Geometry: see drawing. Coordinates: mm, zero at the bounding-box minimum. Give positions to 0.01 mm unless a question says otherwise; leave off trailing zeros. Write each loop counter-clockwise with the first axis right and the second up, starting at its lowest first coordinate (ties: lowest second). Pieces come first, ordered by that corner, then holes. Notation, with made-up numbers: (-4, 59.25) - (0, 59.25) arc R20 cw to (0, 73.25) - close; hole circle Ø3 at (46.5, -17). An arc over 180 degrees is marked (long way). Use a Markdown table: item, result. Add a question column.
1. Section query C-C, the plane x = 68. Return loops of the section in (y, z) (1 decimal).
2. Section query A-A, the plane x = 6.35. Return loops of the section in (y, z) (1 decimal).
3. Pin query (flat end, axial travel): pin 1 (0.5 mm diameter, centred on y = 3, z = 1, fed in from -X); pin 2 (1 mm diameter, centred on x = 30.5, y = 2.5, fed in from +Z); pin 3 (5 mm diameter, centred on x = 43, y = 1.5, fed in from -Z). Return the tip coordinate at first contact, or that it passes through.
4. Material intervals for probe 1 along Y at (x, z) = (6.35, 5) (1 decimal); probe 2 along X at (y, z) = (5, 3.75); probe 3 along Y at (x, z) = (77, 5) (1 decimal), sorted ascending.
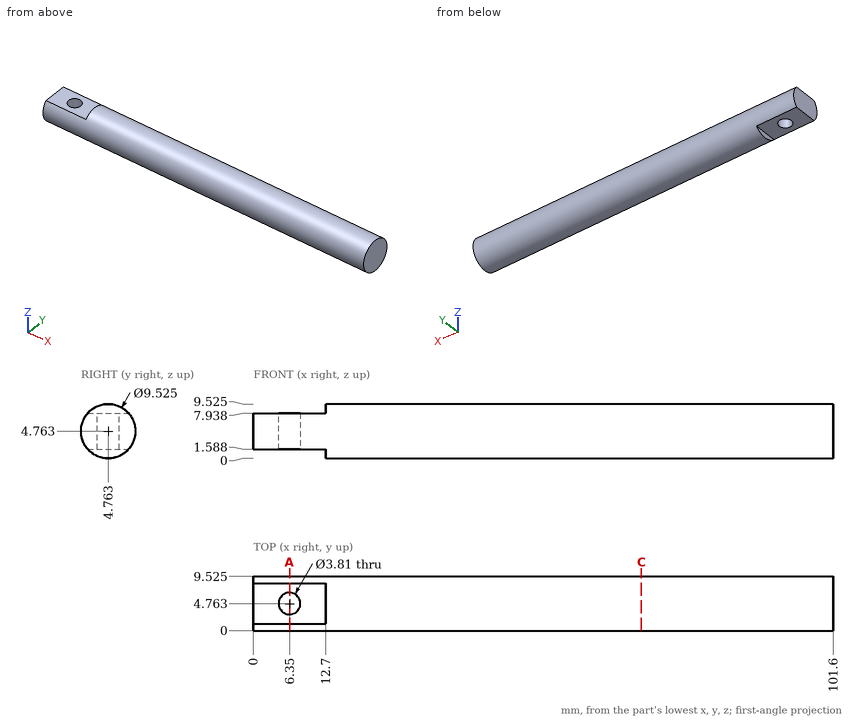
Result sheet:
| question | item | result |
|---|---|---|
| 1 | outline | circle Ø9.5 at (4.8, 4.8) |
| 2 | outline | (1.2, 1.6) - (2.9, 1.6) - (2.9, 7.9) - (1.2, 7.9) arc R4.8 ccw to start; (6.7, 1.6) - (8.3, 1.6) arc R4.8 ccw to (8.3, 7.9) - (6.7, 7.9) - close |
| 3 | pin 1 | stops at x = 12.7 |
| 3 | pin 2 | stops at z = 9.19 |
| 3 | pin 3 | stops at z = 0.06 |
| 4 | probe 1 | y = 0 to 2.9, 6.7 to 9.5 |
| 4 | probe 2 | x = 0 to 4.46, 8.24 to 101.6 |
| 4 | probe 3 | y = 0 to 9.5 |
